Design review of the part built by this model. Coordinates are the model's own, in mm. A direction names the side the tool comes from. Give positions to 0.01 mm unless a question says otherwise; leave off trailing zeros. Loops run counter-clockwise (first coordinate to the right, second up) from the corner with the lowest first, then second, coordinate; pieces in that order, holes last. Notation, with made-up numbers: (-8, 11.25) -> (51, 11.25) arc R22 ccw to (51, 32.25) -> close; hole circle Ø5 at (79.5, 53). An arc over 180 degrees is marked (long way). Answer in a Markdown table with one row per item. Add a question column.
(1) Consider section C-C on y = 7.5. Write out the cut boundary in (x, z).
(2) For line 1 (Y direction, x = -10.5, z = -14.5); line 2 (Y direction, x = -11.5, z = 14.5); line 3 (Z direction, x = -2.5, y = 63), list the stretches that pass through material, from the lowest coordinate up.
(3) For pin 1 (5 mm diameter, centred on y = -3.82, z = 14.5, fed in from +X); pin 2 (7.5 mm diameter, centred on x = 1, y = 27, fed in from +Z); pin 3 (3.5 mm diameter, centred on x = 0.5, y = 99, fed in from -Z), all flat-tipped, find the tip position at first contact; note any pin that passes through.
(4) Consider section A-A on z = -14.5. Write out the cut boundary in (x, y), then the cut area to 3 significant figures.
(5) For faces 1 (the flat face through (0, 49, 9.5)), 2 (the flat face through (9, 0, 6)), 3 (the flat face through (6.5, 99, 0)), 4 (the cylindrical face through (4.38, 1.48, -8.43)), list the 3-axis set-ups (+Z, -Z, +X, -X, +Y, -Y) from which the entire face can be reached by the end or side of a thin tool; tool diameter is ignored.
(6) Consider section B-B on x = -2.5. Write out the cut boundary in (y, z), then the cut area to 3 significant figures.
(7) Consider section D-D on x = -10.75. Write out the cut boundary in (y, z), then the cut area to 3 significant figures.
(8) Draft analysis for pull direction Z (two halves, no side actions). For faces 5 (the cylindrical face through (-10.979, -44.227, 14.695)), 6 (the flat face through (-11, -50, 0)), 7 (the flat face through (0, 49, 12.5)), state which applies: +Z half, -Z half, draft (parallel to the pull), parting line (faces both ways), or undercut.
Autodesk Inventor part; units mm, degrees
ref_plane "YZ Plane" through (0, 0, 0) normal (1, 0, 0) x (0, 1, 0)
ref_plane "XZ Plane" through (0, 0, 0) normal (0, 1, 0) x (-1, 0, 0)
ref_plane "XY Plane" through (0, 0, 0) normal (0, 0, 1) x (1, 0, 0)
sketch "Sketch1" plane through (0, 0, 0) normal (0, 1, 0) x (-1, 0, 0)
  line L0 (-12.5, 12.5) -> (12.5, 12.5)
  line L1 (12.5, 12.5) -> (12.5, -12.5)
  line L2 (12.5, -12.5) -> (-12.5, -12.5)
  line L3 (-12.5, -12.5) -> (-12.5, 12.5)
  line L4 (-12.5, 12.5) -> (12.5, -12.5) construction
  line L5 (12.5, 12.5) -> (-12.5, -12.5) construction
  line L6 (-9.5, 9.5) -> (9.5, 9.5)
  line L7 (9.5, 9.5) -> (9.5, -9.5)
  line L8 (9.5, -9.5) -> (-9.5, -9.5)
  line L9 (-9.5, -9.5) -> (-9.5, 9.5)
  line L10 (-9.5, 9.5) -> (9.5, -9.5) construction
  line L11 (9.5, 9.5) -> (-9.5, -9.5) construction
  point P0 (0, 0)
  dimension "d0" = 25
  dimension "d1" = 25
  dimension "d2" = 3
  dimension "d3" = 3
extrude "Extrusion1" add sketch "Sketch1" along normal blind 100
sketch "Sketch2" plane through (-9.5, 0, 9.5) normal (1, 0, 0) x (0, 0, -1)
  line L0 (0, 0) -> (0, 100)
  line L1 (19, 0) -> (19, 100)
  line L2 (0, 0) -> (0, 100)
  line L3 (19, 0) -> (19, 100)
  line L4 (0, 100) -> (19, 100)
  line L5 (19, 100) -> (19, 97)
  line L6 (19, 97) -> (0, 97)
  line L7 (0, 97) -> (0, 100)
  point P0 (9.5, 0)
  point P1 (0, 97)
  point P2 (19, 97)
  dimension "d6" = 3
extrude "Extrusion2" add sketch "Sketch2" along normal up to surface (19 mm away)
sketch "Sketch3" plane through (0, 100, 0) normal (0, 1, 0) x (1, 0, 0)
  line L0 (9.5, -9.5) -> (9.5, 9.5)
  line L1 (-9.5, -9.5) -> (9.5, -9.5)
  line L2 (-9.5, 9.5) -> (-9.5, -9.5)
  line L3 (9.5, 9.5) -> (-9.5, 9.5)
  line L4 (3.5, 3.5) -> (-3.5, 3.5)
  line L5 (-3.5, 3.5) -> (-3.5, -3.5)
  line L6 (-3.5, -3.5) -> (3.5, -3.5)
  line L7 (3.5, -3.5) -> (3.5, 3.5)
  line L8 (3.5, 3.5) -> (-3.5, -3.5) construction
  line L9 (-3.5, 3.5) -> (3.5, -3.5) construction
  line L10 (6.5, 6.5) -> (-6.5, 6.5)
  line L11 (-6.5, 6.5) -> (-6.5, -6.5)
  line L12 (-6.5, -6.5) -> (6.5, -6.5)
  line L13 (6.5, -6.5) -> (6.5, 6.5)
  line L14 (6.5, 6.5) -> (-6.5, -6.5) construction
  line L15 (-6.5, 6.5) -> (6.5, -6.5) construction
  point P0 (0, 0)
  dimension "d9" = 13
  dimension "d10" = 13
  dimension "d11" = 3
  dimension "d12" = 3
extrude "Extrusion3" cut sketch "Sketch3" against normal blind 200 contours L7 L6 L5 L4 | L13 L12 L11 L10
sketch "Sketch4" plane through (-9.5, 0, 9.5) normal (1, 0, 0) x (0, 0, -1)
  line L0 (0, 0) -> (0, 97)
  line L1 (19, 0) -> (19, 97)
  line L2 (0, 0) -> (19, 0)
  line L3 (19, 0) -> (19, 3)
  line L4 (19, 3) -> (0, 3)
  line L5 (0, 3) -> (0, 0)
  point P0 (9.5, 0)
  dimension "d15" = 3
extrude "Extrusion4" add sketch "Sketch4" along normal up to surface (19 mm away)
sketch "Sketch5" plane through (0, 0, 0) normal (0, -1, 0) x (1, 0, 0)
  line L0 (-6.5, 6.5) -> (6.5, 6.5)
  line L1 (6.5, 6.5) -> (6.5, -6.5)
  line L2 (6.5, -6.5) -> (-6.5, -6.5)
  line L3 (-6.5, -6.5) -> (-6.5, 6.5)
  line L4 (-9.5, -9.5) -> (9.5, -9.5)
  line L5 (9.5, -9.5) -> (9.5, 9.5)
  line L6 (9.5, 9.5) -> (-9.5, 9.5)
  line L7 (-9.5, 9.5) -> (-9.5, -9.5)
  circle A0 centre (0, 0) radius 5
extrude "Extrusion5" cut sketch "Sketch5" against normal blind 200 contours A0
sketch "Sketch9" plane through (0, 0, 0) normal (0, -1, 0) x (1, 0, 0)
  circle A0 centre (0, 0) radius 9.5
  point P0 (0, 0)
extrude "Extrusion9" cut sketch "Sketch9" against normal blind 10
sketch "Sketch10" plane through (0, 0, 0) normal (0, -1, 0) x (1, 0, 0)
  line L0 (12.5, -12.5) -> (-12.5, -12.5)
  line L1 (-12.5, -12.5) -> (-12.5, 12.5)
  line L2 (-12.5, -12.5) -> (-12.5, 12.5)
  line L3 (-12.5, 12.5) -> (-9.5, 12.5)
  line L4 (-9.5, 12.5) -> (-9.5, -12.5)
  line L5 (-9.5, -12.5) -> (-12.5, -12.5)
  line L6 (-12.5, -12.5) -> (-12.5, 12.5)
  line L7 (-6.024, 15.0194) -> (-8.024, 15.0194)
  line L8 (-8.024, -14.9806) -> (-6.024, -14.9806)
  line L9 (-12.5, 12.5) -> (12.5, 12.5)
  line L10 (-12.5, 12.5) -> (-9.5, 12.5)
  line L11 (-9.5, 12.5) -> (-9.5, 17.5)
  line L12 (-9.5, 17.5) -> (-12.5, 17.5)
  line L13 (-12.5, 17.5) -> (-12.5, 12.5)
  line L14 (12.5, -12.5) -> (-12.5, -12.5)
  line L15 (-12.5, -12.5) -> (-9.5, -12.5)
  line L16 (-9.5, -12.5) -> (-9.5, -17.5)
  line L17 (-9.5, -17.5) -> (-12.5, -17.5)
  line L18 (-12.5, -17.5) -> (-12.5, -12.5)
  point P0 (0, 0)
  point P1 (-12.5, 0)
  dimension "d53" = 3
  dimension "d54" = 25
  dimension "d55" = 5
  dimension "d56" = 5
extrude "Extrusion10" add sketch "Sketch10" along normal blind 50
sketch "Sketch11" plane through (-9.5, 0, -12.5) normal (1, 0, 0) x (0, 0, -1)
  line L0 (-30, 0) -> (-30, -50) construction
  line L1 (0, 0) -> (5, 0) construction
  line L2 (-30, -50) -> (5, 0) construction
  line L3 (5, 0) -> (-29.6481, 0) construction
  line L4 (-29.6481, 0) -> (5, -50) construction
  circle A0 centre (-27, -45.7143) radius 1.5
  circle A1 centre (-27, -3.8214) radius 1.5
  circle A2 centre (2, -4.2857) radius 1.5
  circle A3 centre (2, -45.6708) radius 1.5
  line L5 (5, 0) -> (5, -50)
  point P0 (-12.5, 0)
  dimension "d57" = 3
  dimension "d58" = 3
  dimension "d59" = 3
  dimension "d60" = 3
  dimension "d61" = 3
  dimension "d62" = 3
  dimension "d63" = 3
  dimension "d64" = 3
extrude "Extrusion11" cut sketch "Sketch11" against normal through all
properties part number "Cylinder"
Values follow:
| question | item | result |
|---|---|---|
| 1 | outline | (-12.5, -12.5) -> (12.5, -12.5) -> (12.5, 12.5) -> (-12.5, 12.5) -> close; hole (-9.5, -9.5) -> (9.5, -9.5) -> (9.5, 9.5) -> (-9.5, 9.5) -> close |
| 2 | line 1 | -50 to -47.17, -44.17 to -5.79, -2.79 to 0 |
| 2 | line 2 | -50 to -47.21, -44.21 to -5.32, -2.32 to 0 |
| 2 | line 3 | -12.5 to -9.5, 9.5 to 12.5 |
| 3 | pin 1 | x = -9.5 |
| 3 | pin 2 | z = 12.5 |
| 3 | pin 3 | z = -12.5 |
| 4 | outline | (-12.5, -50) -> (-9.5, -50) -> (-9.5, -47.17) -> (-12.5, -47.17) -> close; (-12.5, -44.17) -> (-9.5, -44.17) -> (-9.5, -5.79) -> (-12.5, -5.79) -> close; (-12.5, -2.79) -> (-9.5, -2.79) -> (-9.5, 0) -> (-12.5, 0) -> close |
| 4 | area | 132 mm2 |
| 5 | face 1 | none |
| 5 | face 2 | +Z, -Z, +X, -Y |
| 5 | face 3 | +Y, -Y |
| 5 | face 4 | -Y |
| 6 | outline | (0, -12.5) -> (100, -12.5) -> (100, -6.5) -> (97, -6.5) -> (97, -9.5) -> (3, -9.5) -> (3, -9.17) -> (0, -9.17) -> close; (0, 9.17) -> (3, 9.17) -> (3, 9.5) -> (97, 9.5) -> (97, 6.5) -> (100, 6.5) -> (100, 12.5) -> (0, 12.5) -> close |
| 6 | area | 620 mm2 |
| 7 | outline | (-50, -17.5) -> (0, -17.5) -> (0, -12.5) -> (100, -12.5) -> (100, 12.5) -> (0, 12.5) -> (0, 17.5) -> (-50, 17.5) -> close; hole circle Ø3 at (-45.71, 14.5); hole circle Ø3 at (-45.67, -14.5); hole circle Ø3 at (-4.29, -14.5); hole circle Ø3 at (-3.82, 14.5) |
| 7 | area | 4,220 mm2 |
| 8 | face 5 | undercut |
| 8 | face 6 | draft |
| 8 | face 7 | +Z half |
